Part model, mm, in its own coordinate system. Round coordinates to 2 decimals unless told otherwise and drop trailing zeros. Loops run counter-clockwise (first coordinate to the right, second up) from the corner with the lowest first, then second, coordinate; pieces in that order, holes last.
1) Probe line 1 (X direction, y = -49.5, z = 93.5); line 2 (X direction, y = 24, z = 22). List the from-to ranges inside material, lowest first.
2) Band-saw the part on B-B, the plane x = 34.5. Write the cut outline in (y, z), then the cut area to 3 significant figures.
3) Band-saw the part on C-C, the plane z = 62. Write the cut outline in (x, y), then the cut area to 3 significant figures.
4) Band-saw the part on A-A, the plane y = -28. Write the cut outline in (x, z).
5) Drop flat-ended pins along their axis: P1, Ø1.5, axis at y = 24, z = 28, coming from the -X side; P2, Ø8, axis at y = 23, z = 32.5, coming from the +X side; P3, Ø8, axis at y = -30.5, z = 48, coming from the -X side. Give the stop position or say it passes through.
from build123d import *

# Parameters (mm, degrees)
SKETCH1_W           = 80
SKETCH1_H           = 120
BOSS_EXTRUDE1_DEPTH = 10
BOSS_EXTRUDE2_DEPTH = 60


with BuildPart() as part:
    # Sketch1 → Boss-Extrude1 (new body)
    with BuildSketch(Plane.XY):
        Rectangle(SKETCH1_W, SKETCH1_H)
    extrude(amount=BOSS_EXTRUDE1_DEPTH)

    # Sketch2 → Boss-Extrude2 (add, symmetric)
    with BuildSketch(Plane(origin=(0, 0, 0), x_dir=(1, 0, 0), z_dir=(0, 1, 0))):
        Polygon((40, -10), (-40, -10), (-20, -110), (20, -110), align=None)
    extrude(amount=BOSS_EXTRUDE2_DEPTH, both=True)


solid = part.part
Reported:
1. line 1: x = -23.3 to 23.3
1. line 2: x = -37.6 to 37.6
2. outline: (-60, 0) - (60, 0) - (60, 37.5) - (-60, 37.5) - close
2. area: 4,500 mm2
3. outline: (-29.6, -60) - (29.6, -60) - (29.6, 60) - (-29.6, 60) - close
3. area: 7,100 mm2
4. outline: (-40, 0) - (40, 0) - (40, 10) - (20, 110) - (-20, 110) - (-40, 10) - close
5. P1: stops at x = -36.55
5. P2: stops at x = 36.3
5. P3: stops at x = -33.2
